Read the model definition and answer for the solid it produces. Units are mm, in the model's axes. Give positions to 0.01 mm unless a question says otherwise; leave off trailing zeros. Write each loop counter-clockwise with the first axis right and the second up, starting at its lowest first coordinate (ties: lowest second). Pieces come first, ordered by that corner, then holes. Notation, with made-up numbers: M 54,71.25 L 58,71.25 A16 cw 58,95.25 Z; hole C 26,64 d6. An arc over 180 degrees is marked long. Put each result on its own line as item: value.
from build123d import *

# Parameters (mm, degrees)
F0_W        = 67.9875686765
F0_H        = 50.382964313
F1_DEPTH    = 25.4
F2_T1_DEPTH = 152.4


# Not quite as in the source:
# - a fillet or chamfer that OpenCascade refuses, or shapes differently, is made with other operations: its cross-section is extruded or revolved along the edge and cut away or added


with BuildPart() as f1:
    # F0 (on Front) → F1 (new body)
    with BuildSketch(Plane.XZ):
        with Locations((33.9937843382, 25.1914821565)):
            Rectangle(F0_W, F0_H)
    extrude(amount=F1_DEPTH)

    # F2: fillet of radius 25.4 on 4 edges, made by hand

    # F2_s2 → F2_t1 (cut)
    with BuildSketch(Plane.XZ.offset(-63.5)):
        with BuildLine():
            ThreePointArc((0, 24.982964313), (7.4394877579, 42.9434765552), (25.4, 50.382964313))
            Line((25.4, 50.382964313), (0, 50.382964313))
            Line((0, 50.382964313), (0, 24.982964313))
        make_face()
        with BuildLine():
            ThreePointArc((67.9875686765, 24.982964313), (60.5480809186, 42.9434765552), (42.5875686765, 50.382964313))
            Line((42.5875686765, 50.382964313), (67.9875686765, 50.382964313))
            Line((67.9875686765, 50.382964313), (67.9875686765, 24.982964313))
        make_face()
        with BuildLine():
            ThreePointArc((0, 25.4), (7.4394877579, 7.4394877579), (25.4, 0))
            Line((25.4, 0), (0, 0))
            Line((0, 0), (0, 25.4))
        make_face()
        with BuildLine():
            ThreePointArc((42.5875686765, 0), (60.5480809186, 7.4394877579), (67.9875686765, 25.4))
            Line((67.9875686765, 25.4), (67.9875686765, 0))
            Line((67.9875686765, 0), (42.5875686765, 0))
        make_face()
    extrude(amount=F2_T1_DEPTH, mode=Mode.SUBTRACT)


solid = f1.part
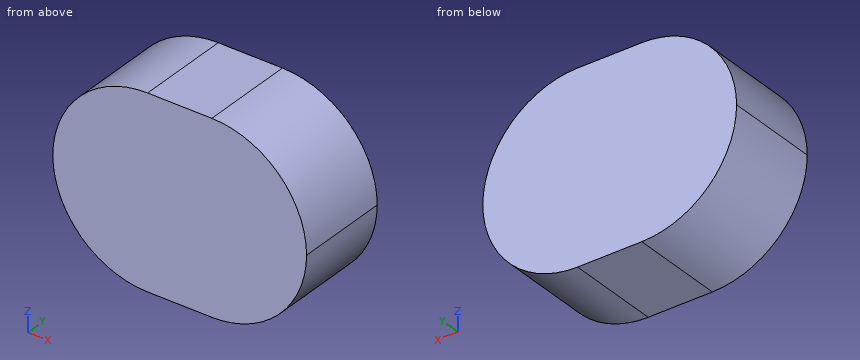
(1) Section A-A on y = -3.75 is taken. Determine the outline of the cut face in (x, z), and give its area (3 significant figures).
Result:
outline: M 0,25.19 A25.4 ccw 25.4,0 L 42.59,0 A25.4 ccw 67.99,25.19 A25.4 ccw 42.59,50.38 L 25.4,50.38 A25.4 ccw Z
area: 2,870 mm²
(2) Given pin 1 Ø4 at (y, z) = (-2.5, 27.5) entering from +X; pin 2 Ø3 at (y, z) = (-20.5, 38) entering from -X; pin 3 Ø4 at (x, y) = (12, -10) entering from +Z, each flat-ended and moving along its own axis, determine where each tip first touches the part or whether it passes through.
Result:
pin 1: stops at x = 67.98
pin 2: stops at x = 2.76
pin 3: stops at z = 47.68
(3) Straight lines are drawn through the part: line 1 along Z through (x, y) = (24.5, -17.75); line 2 along X through (y, z) = (-2, 37); line 3 along Z through (x, y) = (24, -14.5). For each, find the intervals that lie inside material, in ascending order. Write a range as from..to.
Result:
line 1: z = 0.02..50.37
line 2: x = 3.02..64.97
line 3: z = 0.04..50.34
(4) Section B-B on z = 39 is taken. Determine the outline of the cut face in (x, y), and give its area (3 significant figures).
Result:
outline: M 4.22,-25.4 L 63.77,-25.4 L 63.77,0 L 4.22,0 Z
area: 1,510 mm²
(5) Section C-C on x = 13 is taken. Determine the outline of the cut face in (y, z).
Result:
outline: M -25.4,3.23 L 0,3.23 L 0,47.15 L -25.4,47.15 Z
